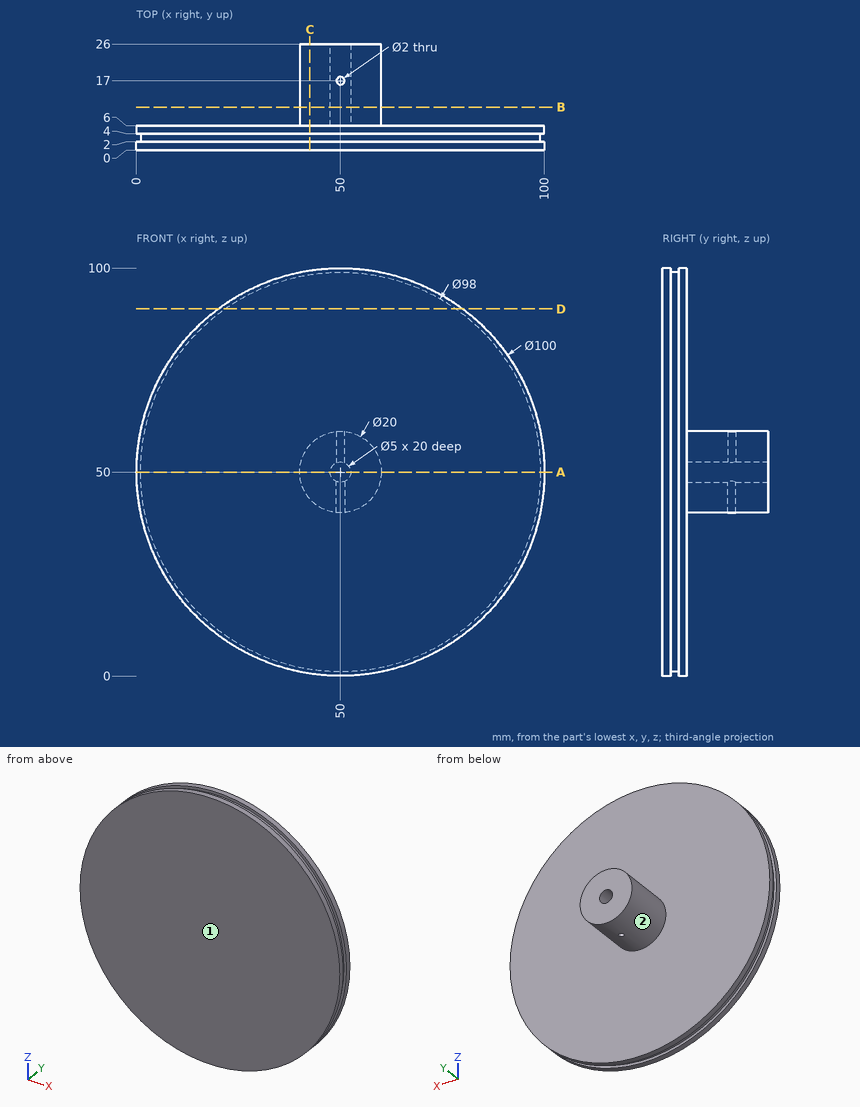
For this review, use the dimensioned drawing (mm, ordinates from the lowest corner) and the shaded views. A direction names the side the tool comes from. Round coordinates to 2 decimals unless told otherwise and drop trailing zeros. Write each loop counter-clockwise with the first axis right and the second up, starting at its lowest first coordinate (ties: lowest second). Pieces come first, ordered by that corner, then holes. Notation, with made-up numbers: (-10.75, -6.75) - (21.25, -6.75) arc R30 cw to (21.25, 21.25) - close; hole circle Ø9 at (20, 89). An arc over 180 degrees is marked (long way). Answer as a JSON object with one key per item and string values.
1. We need section B-B on y = 10.5. Give the boundary of the cut face in (x, z).
Response values:
{"outline": "circle Ø20 at (50, 50); hole circle Ø5 at (50, 50)"}
2. Tool access review of the marked faces 1 and 2: name each direction out of +Z, -Z, +X, -X, +Y, -Y from which nothing blocks a thin tool from reaching the whole face with its end or side.
Response values:
{"face 1": "+Z, -Z, +X, -X, -Y", "face 2": "+Y"}
3. For pin 1 Ø10 at (y, z) = (19, 63.5) entering from -X; pin 2 Ø3 at (x, z) = (26, 27.5) entering from +Y, all flat-tipped, find the tip position at first contact; note any pin that passes through.
Response values:
{"pin 1": "stops at x = 44.73", "pin 2": "stops at y = 6"}
4. We need section C-C on x = 42.5. Give the boundary of the cut face in (y, z).
Response values:
{"outline": "(0, 0.57) - (2, 0.57) - (2, 1.58) - (4, 1.58) - (4, 0.57) - (6, 0.57) - (6, 43.39) - (26, 43.39) - (26, 56.61) - (6, 56.61) - (6, 99.43) - (4, 99.43) - (4, 98.42) - (2, 98.42) - (2, 99.43) - (0, 99.43) - close"}
5. To check wall thickness, follow line 1 along Y through (x, z) = (50, 43.25); line 2 along Z through (x, y) = (50, 19.5); line 3 along X through (y, z) = (17, 43.5). State the ranges of each line that lie inside material, in increasing order.
Response values:
{"line 1": "y = 0 to 16, 18 to 26", "line 2": "z = 40 to 47.5, 52.5 to 60", "line 3": "x = 42.4 to 49, 51 to 57.6"}
6. We need section D-D on z = 90. Give the boundary of the cut face in (x, y).
Response values:
{"outline": "(20, 0) - (80, 0) - (80, 2) - (78.3, 2) - (78.3, 4) - (80, 4) - (80, 6) - (20, 6) - (20, 4) - (21.7, 4) - (21.7, 2) - (20, 2) - close"}
7. We need section A-A on z = 50. Give the boundary of the cut face in (x, y).
Response values:
{"outline": "(0, 0) - (100, 0) - (100, 2) - (99, 2) - (99, 4) - (100, 4) - (100, 6) - (60, 6) - (60, 26) - (52.5, 26) - (52.5, 6) - (47.5, 6) - (47.5, 26) - (40, 26) - (40, 6) - (0, 6) - (0, 4) - (1, 4) - (1, 2) - (0, 2) - close"}
